from build123d import *

# Parameters (mm, degrees)
SKETCH2_W           = 3.25
SKETCH2_H           = 3.25
CUT_EXTRUDE1_DEPTH  = 11
CHAMFER1_SIZE       = 0.5
SKETCH3_R           = 17.5
SKETCH3_R_2         = 15
BOSS_EXTRUDE1_DEPTH = 29
SKETCH4_W           = 3.25
SKETCH4_H           = 3.25
CUT_EXTRUDE2_DEPTH  = 29
CHAMFER2_SIZE       = 0.5


with BuildPart() as part:
    # Sketch1 → Revolve1 (revolve)
    with BuildSketch(Plane.XY, mode=Mode.PRIVATE) as revolve1_sk:
        Polygon((12, 200), (12, 0), (14, 0), (14, 11), (15, 11), (15, 200), align=None)
    revolve(revolve1_sk.sketch.rotate(Axis((0, 0, 0), (0, 1, 0)), 90), axis=Axis((0, 0, 0), (0, 1, 0)))

    # Sketch2 → Cut-Extrude1 (cut)
    with BuildSketch(Plane.XZ):
        with Locations((0, 14)):
            Rectangle(SKETCH2_W, SKETCH2_H)
    extrude(amount=-CUT_EXTRUDE1_DEPTH, mode=Mode.SUBTRACT)

    # Chamfer1
    chamfer1_edges = [part.edges().sort_by_distance(p)[0] for p in [
        (0, 11, 15),
    ]]
    chamfer(chamfer1_edges, length=CHAMFER1_SIZE)

    # Sketch3 → Boss-Extrude1 (add)
    with BuildSketch(Plane(origin=(0, 200, 0), x_dir=(1, 0, 0), z_dir=(0, 1, 0))):
        with Locations(Location((0, 0, 0), (0, 0, 270))):
            Circle(SKETCH3_R)
        with Locations(Location((0, 0, 0), (0, 0, 90))):
            Circle(SKETCH3_R_2, mode=Mode.SUBTRACT)
    extrude(amount=-BOSS_EXTRUDE1_DEPTH)

    # Sketch4 → Cut-Extrude2 (cut)
    with BuildSketch(Plane(origin=(0, 200, 0), x_dir=(1, 0, 0), z_dir=(0, 1, 0))):
        with Locations((0, 17.5)):
            Rectangle(SKETCH4_W, SKETCH4_H)
    extrude(amount=-CUT_EXTRUDE2_DEPTH, mode=Mode.SUBTRACT)

    # Chamfer2
    chamfer2_edges = [part.edges().sort_by_distance(p)[0] for p in [
        (0, 171, 15),
        (-17.481087339, 171, 0.813379038),
        (-17.481087339, 200, 0.813379038),
        (0, 200, 12),
    ]]
    chamfer(chamfer2_edges, length=CHAMFER2_SIZE)


solid = part.part
Input: part model. Units: mm. Frame: model coordinates. A direction names the side the tool comes from. Round coordinates to 2 decimals unless told otherwise and drop trailing zeros. Write each loop counter-clockwise with the first axis right and the second up, starting at its lowest first coordinate (ties: lowest second). Pieces come first, ordered by that corner, then holes.
1) Cut plane C-C (y = 131.5). Return the cut outline in (x, z).
2) Cut plane A-A (z = 0). Return the cut outline in (x, y), then the cut area to 3 significant figures.
3) Draft query along X for faces 1 (the cylindrical face through (-12.65, 92.11, -8.06)), 2 (the flat face through (-7, 171, 14)), 3 (the flat face through (0, 186, -15.875)). Return one class per face: pulls with the +X half, pulls with the -X half, needs draft (parallel to the pull), parting line crosses it, or undercut.
4) Cut plane B-B (y = 179). Return the cut outline in (x, z) (3 decimals).
5) Contact query for flat-ended pins moving along their axis: P1, Ø1.5, axis at y = 80.5, z = -4.5, coming from the -X side; P2, Ø0.8, axis at y = 5, z = 13, coming from the -X side; P3, Ø2.5, axis at x = -0.5, y = 189.5, coming from the -Z side; P4, Ø4, axis at x = -12, y = 107.5, coming from the -Z side. Output: stop coordinate, or through.
6) Ray query, L1, parallel to X at y = 66, z = 0; L2, parallel to X at y = 128.5, z = 3; L3, parallel to Z at x = -5.5, y = 161. Return the intervals inside material, ascending.
7) Reachability of faces 4 (the flat face through (0, 5, 12.375)), 5 (the conical face through (-0.731, 199.858, 17.127)) from +Z, -Z, +X, -X, +Y, -Y: full face, straight path, thin tool, end or side. Return the list, or none.
Geometry says:
1. outline: circle Ø30 at (0, 0); hole circle Ø24 at (0, 0)
2. outline: (-17.5, 171.5) - (-17, 171) - (-15.5, 171) - (-15, 170.5) - (-15, 11.5) - (-14.5, 11) - (-14, 11) - (-14, 0) - (-12, 0) - (-12, 199.5) - (-12.5, 200) - (-17, 200) - (-17.5, 199.5) - close; (12, 0) - (14, 0) - (14, 11) - (14.5, 11) - (15, 11.5) - (15, 170.5) - (15.5, 171) - (17, 171) - (17.5, 171.5) - (17.5, 199.5) - (17, 200) - (12.5, 200) - (12, 199.5) - close
2. area: 1,320 mm2
3. face 1: parting line crosses it
3. face 2: needs draft
3. face 3: undercut
4. outline: (-1.625, -17.424) - (-1.625, -15.875) - (1.625, -15.875) - (1.625, -17.424) arc R17.5 ccw (long way) to start; hole circle Ø24 at (0, 0)
5. P1: stops at x = -14.52
5. P2: stops at x = -6.1
5. P3: stops at z = -17.42
5. P4: stops at z = -11.18
6. L1: x = -15 to -12, 12 to 15
6. L2: x = -14.7 to -11.62, 11.62 to 14.7
6. L3: z = -13.96 to -10.67, 10.67 to 13.96
7. face 4: +Z, -Y
7. face 5: +Y
